Autodesk Inventor part; units mm, degrees
ref_plane "YZ Plane" through (0, 0, 0) normal (1, 0, 0) x (0, 1, 0)
ref_plane "XZ Plane" through (0, 0, 0) normal (0, 1, 0) x (-1, 0, 0)
ref_plane "XY Plane" through (0, 0, 0) normal (0, 0, 1) x (1, 0, 0)
sketch "Sketch1" plane through (0, 0, 0) normal (0, 0, 1) x (1, 0, 0)
  line L0 (0, 0) -> (-128, 0)
  line L1 (-128, 86) -> (0, 86)
  line L2 (0, 86) -> (0, 0)
  line L3 (-128, 71) -> (-138, 61)
  line L4 (-138, 61) -> (-138, 19)
  line L5 (-138, 19) -> (-128, 9)
  line L6 (-128, 0) -> (-128, 9)
  line L7 (-128, 71) -> (-128, 86)
  line L8 (-52, 9) -> (-44, 9)
  line L9 (-44, 9) -> (-44, 3)
  line L10 (-44, 3) -> (-52, 3)
  line L11 (-52, 3) -> (-52, 9)
  line L12 (-52, 77) -> (-44, 77)
  line L13 (-44, 77) -> (-44, 71)
  line L14 (-44, 71) -> (-52, 71)
  line L15 (-52, 71) -> (-52, 77)
  line L16 (-16, 77) -> (-8, 77)
  line L17 (-8, 77) -> (-8, 71)
  line L18 (-8, 71) -> (-16, 71)
  line L19 (-16, 71) -> (-16, 77)
  line L20 (-16, 9) -> (-8, 9)
  line L21 (-8, 9) -> (-8, 3)
  line L22 (-8, 3) -> (-16, 3)
  line L23 (-16, 3) -> (-16, 9)
  line L24 (-34, 83) -> (-26, 83)
  line L25 (-26, 83) -> (-26, 77)
  line L26 (-26, 77) -> (-34, 77)
  line L27 (-34, 77) -> (-34, 83)
  line L28 (-6, 49.9411) -> (-6, 30.0589)
  line L29 (-6, 30.0589) -> (-20.0589, 16)
  line L30 (-20.0589, 16) -> (-39.9411, 16)
  line L31 (-39.9411, 16) -> (-54, 30.0589)
  line L32 (-54, 30.0589) -> (-54, 49.9411)
  line L33 (-54, 49.9411) -> (-39.9411, 64)
  line L34 (-39.9411, 64) -> (-20.0589, 64)
  line L35 (-20.0589, 64) -> (-6, 49.9411)
  line L36 (-51, 61) -> (-9, 61) construction
  line L37 (-9, 61) -> (-9, 19) construction
  line L38 (-9, 19) -> (-51, 19) construction
  line L39 (-51, 19) -> (-51, 61) construction
  circle A0 centre (-51, 61) radius 3.2
  circle A1 centre (-51, 19) radius 3.2
  circle A2 centre (-9, 19) radius 3.2
  circle A3 centre (-9, 61) radius 3.2
  circle A4 centre (-131, 60) radius 2.75
  circle A5 centre (-131, 20) radius 2.75
  line L40 (-124, 77) -> (-116, 77)
  line L41 (-116, 77) -> (-116, 71)
  line L42 (-116, 71) -> (-124, 71)
  line L43 (-124, 71) -> (-124, 77)
  line L44 (-124, 9) -> (-116, 9)
  line L45 (-116, 9) -> (-116, 3)
  line L46 (-116, 3) -> (-124, 3)
  line L47 (-124, 3) -> (-124, 9)
  line L48 (-121, 63) -> (-113, 63)
  line L49 (-113, 63) -> (-113, 57)
  line L50 (-113, 57) -> (-121, 57)
  line L51 (-121, 57) -> (-121, 63)
  line L52 (-121, 23) -> (-113, 23)
  line L53 (-113, 23) -> (-113, 17)
  line L54 (-113, 17) -> (-121, 17)
  line L55 (-121, 17) -> (-121, 23)
  circle A6 centre (-66, 67) radius 2.75
  circle A7 centre (-66, 13) radius 2.75
  line L56 (-60, 86) -> (-60, 0) construction
  line L57 (-132, 67) -> (-60, 67) construction
  line L58 (-132, 13) -> (-60, 13) construction
  line L59 (-83, 63) -> (-75, 63)
  line L60 (-75, 63) -> (-75, 57)
  line L61 (-75, 57) -> (-83, 57)
  line L62 (-83, 57) -> (-83, 63)
  line L63 (-83, 23) -> (-75, 23)
  line L64 (-75, 23) -> (-75, 17)
  line L65 (-75, 17) -> (-83, 17)
  line L66 (-83, 17) -> (-83, 23)
  line L67 (-73, 77) -> (-65, 77)
  line L68 (-65, 77) -> (-65, 71)
  line L69 (-65, 71) -> (-73, 71)
  line L70 (-73, 71) -> (-73, 77)
  line L71 (-73, 9) -> (-65, 9)
  line L72 (-65, 9) -> (-65, 3)
  line L73 (-65, 3) -> (-73, 3)
  line L74 (-73, 3) -> (-73, 9)
  line L75 (-113, 83) -> (-105, 83)
  line L76 (-105, 83) -> (-105, 77)
  line L77 (-105, 77) -> (-113, 77)
  line L78 (-113, 77) -> (-113, 83)
  line L79 (-84, 83) -> (-76, 83)
  line L80 (-76, 83) -> (-76, 77)
  line L81 (-76, 77) -> (-84, 77)
  line L82 (-84, 77) -> (-84, 83)
  circle A8 centre (-106, 40) radius 2.75
  circle A9 centre (-74, 40) radius 2.75
  point P0 (-30, 40)
  point P1 (-138, 40)
  point P2 (-54, 40)
  point P3 (-51, 40)
  point P4 (-30, 61)
  point P5 (-30, 64)
  dimension "d1" = 45
  dimension "d2" = 10
  dimension "d3" = 6
  dimension "d4" = 6
  dimension "d5" = 3
  dimension "d6" = 8
  dimension "d7" = 8
  dimension "d8" = 6
  dimension "d10" = 3
  dimension "d11" = 48
  dimension "d12" = 8
  dimension "d13" = 6
  dimension "d14" = 42
  dimension "d15" = 42
  dimension "d16" = 6.4
  dimension "d17" = 6.4
  dimension "d18" = 6.4
  dimension "d19" = 6.4
  dimension "d20" = 5.5
  dimension "d21" = 5.5
  dimension "d22" = 7
  dimension "d23" = 11
  dimension "d24" = 11
  dimension "d25" = 6
  dimension "d26" = 8
  dimension "d27" = 6
  dimension "d28" = 6
  dimension "d29" = 8
  dimension "d30" = 6
  dimension "d31" = 8
  dimension "d32" = 8
  dimension "d33" = 5.5
  dimension "d34" = 5.5
  dimension "d35" = 4
  dimension "d36" = 4
  dimension "d37" = 8
  dimension "d38" = 8
  dimension "d39" = 8
  dimension "d40" = 4
  dimension "d41" = 8
  dimension "d42" = 128
  dimension "d43" = 68
  dimension "d44" = 8
  dimension "d45" = 43
  dimension "d47" = 10
  dimension "d48" = 15
  dimension "d49" = 62
  dimension "d50" = 10
  dimension "d52" = 8
  dimension "d53" = 3
  dimension "d54" = 8
  dimension "d55" = 3
  dimension "d56" = 5.5
  dimension "d57" = 5.5
  dimension "d58" = 14
  dimension "d59" = 32
  dimension "d65" = 34
extrude "Extrusion1" add sketch "Sketch1" along normal blind 6
chamfer "Chamfer1" distance 2 angle 45 4 edges at (-128, 0, 3) (-128, 86, 3) (0, 86, 3) (0, 0, 3)
properties part number "x_iddler_bottom"
Input: part model. Units: mm. Frame: model coordinates. A direction names the side the tool comes from. Coordinates: 2 decimals unless noted, no trailing zeros. Loops run counter-clockwise (first coordinate to the right, second up) from the corner with the lowest first, then second, coordinate; pieces in that order, holes last. Notation, with made-up numbers: M 6,50 L 22,50 A30 cw 22,73 Z; hole C 81,89 d7. An arc over 180 degrees is marked long. Answer in a Markdown table with one row per item.
1. Section A-A, the plane x = -131. Output: boundary loops of the cut face in (y, z), then the cut area to 3 significant figures.
Response:
| item | result |
|---|---|
| outline | M 12,0 L 17.25,0 L 17.25,6 L 12,6 Z; M 22.75,0 L 57.25,0 L 57.25,6 L 22.75,6 Z; M 62.75,0 L 68,0 L 68,6 L 62.75,6 Z |
| area | 270 mm2 |
2. Reachability of faces 1 (the flat face through (-12.93, 23.13, 2.96)), 2 (the flat face through (-133, 14, 3)) from +Z, -Z, +X, -X, +Y, -Y: full face, straight path, thin tool, end or side. Return the list, or none.
Response:
| item | result |
|---|---|
| face 1 | +Z, -Z |
| face 2 | +Z, -Z, -X, -Y |
3. First-contact query: pin 1 (2 mm diameter, centred on y = 14.5, z = 1.5, fed in from -X); pin 2 (1.8 mm diameter, centred on y = 75, z = 3, fed in from -X); pin 3 (1 mm diameter, centred on y = 63, z = 1, fed in from -X). Flat tips, straight axial feed; report the tip coordinate or a pass-through.
Response:
| item | result |
|---|---|
| pin 1 | stops at x = -134.5 |
| pin 2 | stops at x = -128 |
| pin 3 | stops at x = -136.5 |
4. Material intervals for line 1 (X direction, y = 5.5, z = 2); line 2 (Y direction, x = -69, z = 1.55); line 3 (X direction, y = 36.5, z = 3.05), sorted ascending.
Response:
| item | result |
|---|---|
| line 1 | x = -128 to -124, -116 to -73, -65 to -52, -44 to -16, -8 to 0 |
| line 2 | y = 0 to 3, 9 to 71, 77 to 86 |
| line 3 | x = -138 to -54, -6 to 0 |
5. Section C-C, the plane x = -24. Output: boundary loops of the cut face in (y, z), then the cut area to 3 significant figures.
Response:
| item | result |
|---|---|
| outline | M 0,0 L 16,0 L 16,6 L 0,6 Z; M 64,0 L 86,0 L 86,6 L 64,6 Z |
| area | 228 mm2 |
6. Section B-B, the plane y = 45.5. Output: boundary loops of the cut face in (x, z).
Response:
| item | result |
|---|---|
| outline | M -138,0 L -54,0 L -54,6 L -138,6 Z; M -6,0 L 0,0 L 0,6 L -6,6 Z |
7. Draft query along Y for faces 3 (the flat face through (-48, 77, 3)), 4 (the flat face through (-133, 66, 3)), 5 (the flat face through (-128, 77, 3)). Return one class per face: pulls with the +Y half, pulls with the -Y half, needs draft (parallel to the pull), parting line crosses it, or undercut.
Response:
| item | result |
|---|---|
| face 3 | undercut |
| face 4 | pulls with the +Y half |
| face 5 | needs draft |
8. Section D-D, the plane z = 2.85. Count the separate pieces of the cut face and the enclosed holes in it, then the cut area to 3 significant figures.
Response:
| item | result |
|---|---|
| separate pieces | 1 |
| enclosed holes | 26 |
| area | 8,620 mm2 |
